```python
from build123d import *

# Parameters (mm, degrees)
F0_R            = 40.8
F1_DEPTH        = 8
F4_R            = 3.15
F6_W            = 4.8
F6_H            = 38.4
F7_DEPTH        = 8.001
F9_DEPTH        = 8
F10_R           = 11.5
F10_R_2         = 1.6
F11_DEPTH       = 8.001
F13_D           = 3.3
F13_CBORE_D     = 6.5
F13_CBORE_DEPTH = 6


# Not quite as in the source:
# - a feature names something its author has since deleted; it is built from what else it names


with BuildPart() as f1:
    # F0 (on Top) → F1 (new body)
    with BuildSketch(Plane.XY):
        Circle(F0_R)
    extrude(amount=F1_DEPTH)

    # F2 (on Right) → F3 (revolve, cut)
    with BuildSketch(Plane.YZ):
        Polygon((0, 8), (0, 0), (9.525, 0), (9.525, 6), (7.25, 6), (7.25, 8), align=None)
    revolve(axis=Axis((0, 0, 10.7360328796), (0, 0, 1)), mode=Mode.SUBTRACT)

    # F4 (on Right) → F5 (revolve, cut)
    with BuildSketch(Plane.YZ):
        with Locations((31, 9)):
            Circle(F4_R)
    revolve(axis=Axis((0, 0, 6.3867427816), (0, 0, 1)), mode=Mode.SUBTRACT)

    # F6 (on Top) → F7 (cut, through all)
    with BuildSketch(Plane.XY):
        with Locations((-38.4, 0)):
            Rectangle(F6_W, F6_H)
    extrude(amount=F7_DEPTH, mode=Mode.SUBTRACT)

    # F8 (on Top) → F9 (join, through all)
    with BuildSketch(Plane.XY):
        with BuildLine():
            Line((-94.75, 20.7850348986), (-94.75, -20.7850348986))
            Line((-94.75, -20.7850348986), (-8.8307362487, -39.8328770905))
            ThreePointArc((-8.8307362487, -39.8328770905), (-24.6754459414, -32.4924970969), (-36, -19.2))
            Line((-36, -19.2), (-36, 19.2))
            ThreePointArc((-36, 19.2), (-24.6754459414, 32.4924970969), (-8.8307362487, 39.8328770905))
            Line((-8.8307362487, 39.8328770905), (-94.75, 20.7850348986))
        make_face()
    extrude(amount=F9_DEPTH)

    # F10 (on face) → F11 (cut, through all)
    with BuildSketch(Plane.XY.offset(8)):
        with Locations((-56.25, 0)):
            Circle(F10_R)
        with Locations((-92.25, 17.7850348986)):
            Circle(F10_R_2)
        with Locations((-92.25, -17.7850348986)):
            Circle(F10_R_2)
        with BuildLine():
            Line((-55.2488153952, 23.5201616153), (-56.2488153952, 23.5201616153))
            ThreePointArc((-56.2488153952, 23.5201616153), (-57.848786069, 21.9104743704), (-56.2294412604, 20.3202789187))
            Line((-56.2294412604, 20.3202789187), (-55.2488153952, 20.3202789187))
            ThreePointArc((-55.2488153952, 20.3202789187), (-53.6488740469, 21.920220267), (-55.2488153952, 23.5201616153))
        make_face()
        with BuildLine():
            Line((-77.1680206657, 1.6075620275), (-78.1680206657, 1.6075620275))
            ThreePointArc((-78.1680206657, 1.6075620275), (-79.7679913396, 0.0172492724), (-78.1873948004, -1.5923206691))
            Line((-78.1873948004, -1.5923206691), (-77.1680206657, -1.5923206691))
            ThreePointArc((-77.1680206657, -1.5923206691), (-75.5680793174, 0.0076206792), (-77.1680206657, 1.6075620275))
        make_face()
        with BuildLine():
            Line((-55.2488164927, -20.3202952302), (-56.2488164927, -20.3202952302))
            ThreePointArc((-56.2488164927, -20.3202952302), (-57.8487871666, -21.9299824752), (-56.229442358, -23.5201779268))
            Line((-56.229442358, -23.5201779268), (-55.2488164927, -23.5201779268))
            ThreePointArc((-55.2488164927, -23.5201779268), (-53.6488751444, -21.9202365785), (-55.2488164927, -20.3202952302))
        make_face()
    extrude(amount=-F11_DEPTH, mode=Mode.SUBTRACT)

    # F13 (through all)
    with Locations(Plane.XY.offset(8)):
        with Locations((-40.5, 24), (-40.5, -24), (37.5, 0)):
            CounterBoreHole(F13_D / 2, F13_CBORE_D / 2, F13_CBORE_DEPTH)


solid = f1.part
```
Input: part model. Units: mm. Frame: model coordinates. A direction names the side the tool comes from. Give positions to 0.01 mm unless a question says otherwise; leave off trailing zeros. Order: outer loops, then holes, each group sorted by start corner. A loop starts at its lowest first (then second) coordinate and runs counter-clockwise, first axis right, second up.
1. Section D-D on x = -64.5. Return the cut outline in (y, z), and give its area (3 significant figures).
Derived:
outline: (-27.49, 0) - (-8.01, 0) - (-8.01, 8) - (-27.49, 8) - close; (8.01, 0) - (27.49, 0) - (27.49, 8) - (8.01, 8) - close
area: 312 mm2
2. Section A-A on x = -48.5. Return the cut outline in (y, z).
Derived:
outline: (-31.04, 0) - (-8.5, 0) - (-8.5, 8) - (-31.04, 8) - close; (8.5, 0) - (31.04, 0) - (31.04, 8) - (8.5, 8) - close
3. Reachability of faces 1 (the flat face through (6, -6, 8)), 2 (the flat face through (-42, -23, 2)), 3 (the cylindrical face through (-57.85, -21.89, 4.06)), 4 (the cylindrical face through (5.796, -7.559, 3.042)) from +Z, -Z, +X, -X, +Y, -Y: full face, straight path, thin tool, end or side. Return the list, or none.
Derived:
face 1: +Z, +X, -X, +Y, -Y
face 2: +Z
face 3: +Z, -Z
face 4: -Z
4. Material intervals for L1, parallel to Y at x = -92.25, z = 5.25; L2, parallel to Y at x = -40.5, z = 3.55; L3, parallel to X at y = 2, z = 1.5, sorted ascending.
Derived:
L1: y = -21.34 to -19.39, -16.19 to 16.19, 19.39 to 21.34
L2: y = -32.81 to -27.25, -20.75 to 20.75, 27.25 to 32.81
L3: x = -94.75 to -67.57, -44.93 to -9.31, 9.31 to 40.75
5. Section B-B on y = 0. Give the number of separate pieces and of enclosed holes in the cut face, and give its area (3 significant figures).
Derived:
separate pieces: 5
enclosed holes: 0
area: 659 mm2
6. Mould query, pull axis X, two halves, no side actions, for faces 5 (the flat face through (-28, 1, 0)), 6 (the flat face through (36, 1, 2)). Classes: released by +X, released by -X, zero draft, split by the parting line, or undercut.
Derived:
face 5: zero draft
face 6: undercut
7. Pin query (flat end, axial travel): pin 1 (2 mm diameter, centred on x = 37.5, y = 0, fed in from -Z); pin 2 (1.1 mm diameter, centred on x = -55.5, z = 4, fed in from +Y); pin 3 (0.8 mm diameter, centred on x = -55.5, z = 2.5, fed in from -Y); pin 4 (3 mm diameter, centred on x = -41, y = 25, fed in from +Z). Return the tip coordinate at first contact, or that it passes through.
Derived:
pin 1: passes through
pin 2: stops at y = 29.61
pin 3: stops at y = -29.58
pin 4: stops at z = 2
8. Section C-C on x = -92.25. Return the cut outline in (y, z), and give its area (3 significant figures).
Derived:
outline: (-21.34, 0) - (-19.39, 0) - (-19.39, 8) - (-21.34, 8) - close; (-16.19, 0) - (16.19, 0) - (16.19, 8) - (-16.19, 8) - close; (19.39, 0) - (21.34, 0) - (21.34, 8) - (19.39, 8) - close
area: 290 mm2
